Could you check a few things on this drawing? It's one solid part, dimensions in mm from its lowest x, y, z. A direction names the side the tool comes from. Give positions to 0.01 mm unless a question says otherwise; leave off trailing zeros. Loops run counter-clockwise (first coordinate to the right, second up) from the corner with the lowest first, then second, coordinate; pieces in that order, holes last. Notation, with made-up numbers: M -36,25 L -20,25 A12 ccw -20,30 Z; hole C -31,48 d4. An arc over 180 degrees is marked long. Return JSON: item names as keys, results as strings. Group by question number.
1. If we section it at B-B (y = 12.5): Write out the boundary of the cut face in (x, z) (3 decimals).
2. For the marked faces 1 and 2, which set-ups out of +Z, -Z, +X, -X, +Y, -Y let a thin tool reach every point of the face, with its end or its side?
3. Please list where these lines run through material, in increasing order: line 1 (Y direction, x = 53.2, z = 63.5) (3 decimals); line 2 (X direction, y = 4.25, z = 94.5) (3 decimals); line 3 (Y direction, x = 13, z = 34) (3 decimals).
4. If we section it at A-A (z = 63.5): Write out the boundary of the cut face in (x, y) (3 decimals), plus the area to 3 significant figures.
5. If we section it at D-D (x = 48): Write out the boundary of the cut face in (y, z) (3 decimals).
6. For pin 1 (3 mm diameter, centred on x = 21, z = 99, fed in from +Y) (3 decimals); pin 2 (10 mm diameter, centred on x = 48, z = 85, fed in from +Y) (3 decimals); pin 3 (12 mm diameter, centred on x = 10, y = 13, fed in from +Z); pin 4 (14.5 mm diameter, centred on y = 15.875, z = 63.5, fed in from -X), each with a flat end and sliding along its axis, tell me the tip position at first contact or that it passes through.
7. If we section it at C-C (z = 17): Write out the boundary of the cut face in (x, y) (3 decimals).
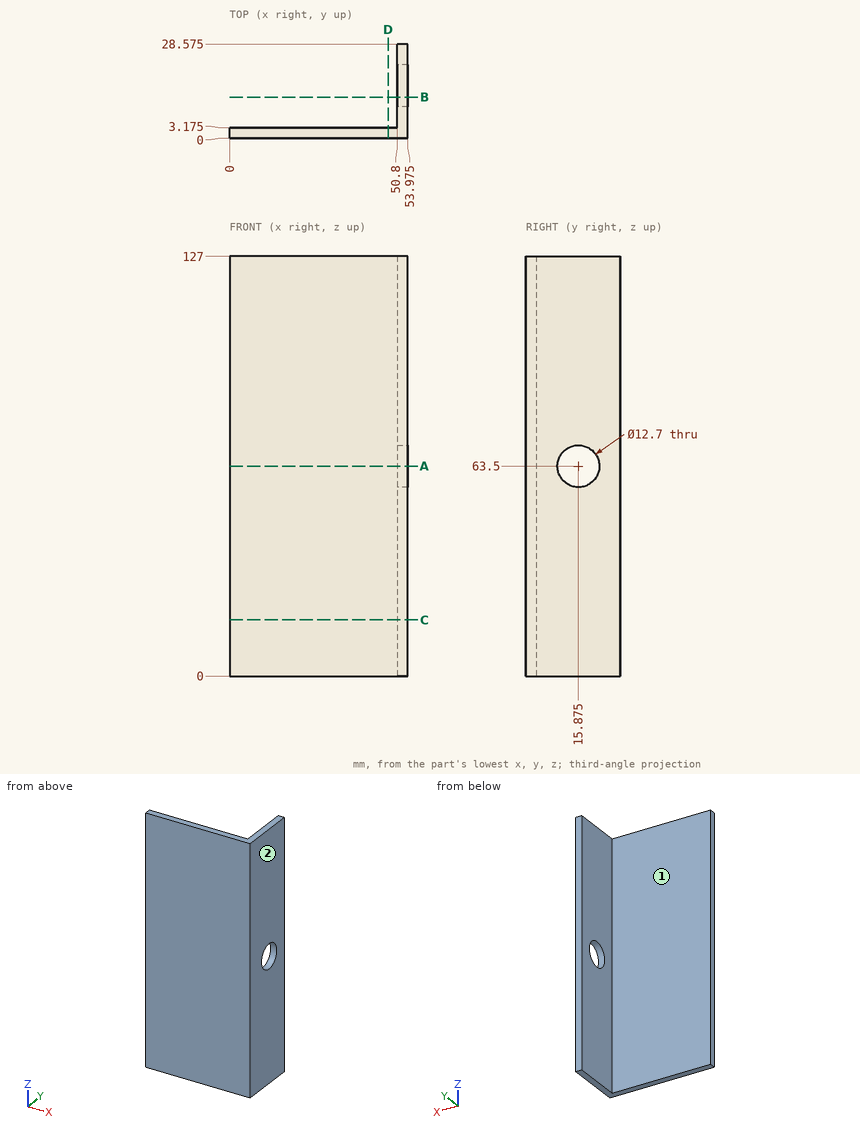
Answer:
{
 "1": {"outline": "M 50.8,0 L 53.975,0 L 53.975,58.121 L 50.8,58.121 Z; M 50.8,68.879 L 53.975,68.879 L 53.975,127 L 50.8,127 Z"},
 "2": {"face 1": "+Z, -Z, -X, +Y", "face 2": "+Z, -Z, +X, +Y, -Y"},
 "3": {"line 1": "y = 0 to 9.525, 22.225 to 28.575", "line 2": "x = 50.8 to 53.975", "line 3": "y = 0 to 3.175"},
 "4": {"outline": "M 0,0 L 53.975,0 L 53.975,9.525 L 50.8,9.525 L 50.8,3.175 L 0,3.175 Z; M 50.8,22.225 L 53.975,22.225 L 53.975,28.575 L 50.8,28.575 Z", "area": "212 mm²"},
 "5": {"outline": "M 0,0 L 3.175,0 L 3.175,127 L 0,127 Z"},
 "6": {"pin 1": "stops at y = 3.175", "pin 2": "stops at y = 28.575", "pin 3": "passes through", "pin 4": "stops at x = 50.8"},
 "7": {"outline": "M 0,0 L 53.975,0 L 53.975,28.575 L 50.8,28.575 L 50.8,3.175 L 0,3.175 Z"}
}
